Can you work these out from the model? Positions are in its coordinate system, mm. Face numbers are marked on the shaded views. A direction names the side the tool comes from. Coordinates: 2 decimals unless noted, no trailing zeros. Loops run counter-clockwise (first coordinate to the right, second up) from the corner with the lowest first, then second, coordinate; pieces in that order, holes last.
Autodesk Inventor part; units mm, degrees
ref_plane "Work Plane1" through (0, 0, 0) normal (0, 1, 0) x (1, 0, 0)
ref_plane "YZ Plane" through (0, 0, 0) normal (1, 0, 0) x (0, 1, 0)
ref_plane "XZ Plane" through (0, 0, 0) normal (0, 1, 0) x (-1, 0, 0)
sketch "Sketch1" plane through (0, 0, 0) normal (0, 1, 0) x (-1, 0, 0)
  line L0 (17.0879, 31.457) -> (-17.8371, 31.457)
  line L1 (-17.8371, 31.457) -> (-17.8371, -31.3318)
  line L2 (-17.8371, -31.3318) -> (17.0879, -31.3318)
  line L3 (17.0879, -31.3318) -> (17.0879, 31.457)
  point P0 (0, 0)
  dimension "d0" = 34.925
  dimension "d1" = 62.7888
extrude "Extrusion1" add sketch "Sketch1" along normal blind 9.7028
sketch "Sketch2" plane through (0, 9.7028, 0) normal (0, 1, 0) x (1, 0, 0)
  line L0 (17.8371, -31.457) -> (17.8371, 31.3318)
  line L1 (-17.0879, 31.3318) -> (-17.0879, -31.457)
  line L2 (17.8371, 31.3318) -> (-17.0879, 31.3318)
  line L3 (-17.0879, 31.3318) -> (-17.0879, 21.1718)
  line L4 (-17.0879, 21.1718) -> (17.8371, 21.1718)
  line L5 (17.8371, 21.1718) -> (17.8371, 31.3318)
  point P0 (0, 0)
  dimension "d4" = 10.16
extrude "Extrusion2" add sketch "Sketch2" along normal blind 11.049
sketch "Sketch3" plane through (0, 0, 0) normal (0, -1, 0) x (1, 0, 0)
  line L0 (17.8371, -31.3318) -> (-17.0879, -31.3318)
  line L1 (-17.0879, -31.3318) -> (-17.0879, -25.0072)
  line L2 (-17.0879, -31.3318) -> (-17.0879, 31.457)
  line L3 (-17.0879, -25.0072) -> (-3.5751, -25.0072)
  line L4 (-3.5751, -25.0072) -> (-3.5751, -18.962)
  line L5 (-3.5751, -18.962) -> (-3.2703, -18.962)
  line L6 (-3.2703, -18.962) -> (-3.2703, 10.883)
  line L7 (-3.2703, 10.883) -> (-3.5751, 10.883)
  line L8 (-3.5751, 10.883) -> (-3.5751, 16.9282)
  line L9 (-3.5751, 16.9282) -> (-16.9609, 16.9282)
  line L10 (-16.9609, 16.9282) -> (-17.0879, 16.9282)
  point P0 (0, 0)
  dimension "d7" = 6.3246
  dimension "d8" = 13.5128
  dimension "d9" = 6.0452
  dimension "d10" = 0.3048
  dimension "d11" = 29.845
  dimension "d14" = 0.3048
  dimension "d15" = 6.0452
  dimension "d16" = 13.3858
extrude "Extrusion3" cut sketch "Sketch3" against normal blind 2.794
sketch "Sketch4" plane through (0, 2.794, 0) normal (0, -1, 0) x (1, 0, 0)
  line L0 (-3.5751, 16.9282) -> (-17.0879, 16.9282)
  line L1 (-17.0879, 16.9282) -> (-17.0879, 10.883)
  line L2 (-17.0879, 10.883) -> (-3.5751, 10.883)
  line L3 (-3.5751, 10.883) -> (-3.5751, 16.9282)
  point P0 (0, 0)
  dimension "d19" = 13.5128
  dimension "d20" = 6.0452
sketch "Sketch5" plane through (0, 2.794, 0) normal (0, -1, 0) x (1, 0, 0)
  line L0 (-3.5751, -18.962) -> (-3.5751, -25.0072)
  line L1 (-3.5751, -25.0072) -> (-17.0879, -25.0072)
  line L2 (-17.0879, -25.0072) -> (-17.0879, -18.962)
  line L3 (-17.0879, -18.962) -> (-3.5751, -18.962)
  line L4 (-3.5751, -18.962) -> (-3.5751, -25.0072)
  point P0 (0, 0)
  dimension "d21" = 13.5128
  dimension "d22" = 6.0452
extrude "Extrusion5" add sketch "Sketch4" along normal blind 1.5748
extrude "Extrusion6" add sketch "Sketch5" along normal blind 1.5748
sketch "Sketch6" plane through (0, 9.7028, 0) normal (0, 1, 0) x (1, 0, 0)
  circle A0 centre (-11.6221, -2.8625) radius 7.9629
  line L0 (-17.0879, 18.962) -> (-17.0879, -10.883)
  line L1 (-11.6221, -10.1806) -> (-11.6221, 5.913) construction
  line L2 (-14.7946, -10.1806) -> (-14.7946, 5.913)
  line L3 (-8.4496, 5.913) -> (-8.4496, -10.1806)
  arc A1 (-8.4496, 5.913) -> (-14.7946, 5.913) centre (-11.6221, 5.913) ccw
  point P0 (0, 0)
  point P1 (-17.0879, 21.1718)
  point P2 (-11.6221, -2.1338)
  point P3 (-17.0879, 2.9283)
  point P4 (-17.0879, -8.6532)
  point P5 (-8.4496, 4.4412)
  point P6 (-14.7946, 4.4412)
  dimension "d31" = 15.9258
extrude "Extrusion7" cut sketch "Sketch6" against normal blind 25.4 contours A0 L3 | L3 A0 L2 | A0 L2 A1 L3 | L2 A0 L0
ref_plane "Work Plane1" through (0, 0, 0) normal (0, 1, 0) x (1, 0, 0)
sketch "Sketch7" plane through (0, 9.7028, 0) normal (0, 1, 0) x (1, 0, 0)
  line L0 (17.8371, -31.457) -> (17.8371, -28.663)
  line L1 (17.8371, -28.663) -> (17.8371, -26.4532)
  line L2 (14.7637, -26.4532) -> (12.5539, -26.4532)
  circle A0 centre (12.5539, -26.4532) radius 2.2098
  circle A1 centre (12.5539, -5.168) radius 2.2098
  line L3 (-17.0879, -8.6532) -> (-17.0879, -31.457)
  line L4 (-17.0879, -26.4532) -> (-13.7859, -26.4532) construction
  circle A2 centre (-11.5761, -26.4532) radius 2.2098
  line L5 (-11.5761, -14.7184) -> (-11.5761, -13.4484)
  circle A3 centre (-11.5761, -13.4484) radius 1.27
  line L6 (-11.5761, -13.4484) -> (-17.0879, -13.4484)
  line L7 (-17.0879, -16.9282) -> (-17.0879, -10.883)
  circle A4 centre (12.5539, -5.168) radius 4.1148
  circle A5 centre (12.5539, -26.4532) radius 4.1148
  circle A6 centre (-11.5761, -26.4532) radius 4.1148
  point P0 (0, 0)
  dimension "d37" = 2.794
  dimension "d38" = 2.2098
  dimension "d39" = 3.0734
  dimension "d40" = 2.2098
  dimension "d42" = 4.4196
  dimension "d43" = 4.4196
  dimension "d47" = 4.4196
  dimension "d49" = 1.27
  dimension "d50" = 2.54
  dimension "d58" = 8.2296
  dimension "d59" = 8.2296
  dimension "d60" = 8.2296
extrude "Extrusion8" cut sketch "Sketch7" against normal blind 25.4 contours A0 | A1 | A2 | A3 L6 L5 | L5 L6 A3
sketch "Sketch9" plane through (0, 1.2192, 0) normal (0, -1, 0) x (1, 0, 0)
  line L0 (-3.5751, -18.962) -> (-17.0879, -18.962)
  line L1 (-17.0879, -18.962) -> (-11.5761, -18.962)
  line L2 (-11.5761, -25.0595) -> (-11.5761, -21.2495)
  circle A0 centre (-11.5761, -21.2495) radius 1.27
  point P0 (0, 0)
  dimension "d53" = 5.5118
  dimension "d54" = 3.81
  dimension "d55" = 2.54
extrude "Extrusion9" cut sketch "Sketch9" against normal blind 8.4836
sketch "Sketch11" plane through (0, 0, 0) normal (0, -1, 0) x (1, 0, 0)
  circle A0 centre (-11.5761, 26.4532) radius 2.2098
  circle A1 centre (-11.5761, 26.4532) radius 4.1148
  circle A2 centre (12.5539, 26.4532) radius 2.2098
  circle A3 centre (12.5539, 26.4532) radius 4.1148
  circle A4 centre (12.5539, 5.168) radius 2.2098
  circle A5 centre (12.5539, 5.168) radius 4.1148
  point P0 (0, 0)
  dimension "d62" = 8.2296
  dimension "d63" = 8.2296
  dimension "d64" = 8.2296
extrude "Extrusion10" cut sketch "Sketch11" against normal blind 5.6642 contours A0 | A1 | A3 | A5
sketch "Sketch12" plane through (17.8371, 0, -31.3318) normal (0, 0, -1) x (-1, 0, 0)
  line L0 (0, 0) -> (0, 20.7518)
  line L1 (0, 20.7518) -> (13.9446, 20.7518)
  line L2 (0, 20.7518) -> (34.925, 20.7518)
  line L3 (13.9446, 20.7518) -> (17.4117, 20.7518)
  line L4 (17.4117, 20.7518) -> (17.4117, 17.9832)
  line L5 (17.4117, 17.9832) -> (17.4117, 14.5161)
  circle A0 centre (17.4117, 14.5161) radius 2.2479
  circle A1 centre (17.4117, 14.5161) radius 3.4671
  point P0 (17.8371, 0)
  dimension "d67" = 13.9446
  dimension "d68" = 3.4671
  dimension "d69" = 2.7686
  dimension "d70" = 3.4671
  dimension "d71" = 4.4958
  dimension "d72" = 6.9342
extrude "Extrusion11" cut sketch "Sketch12" against normal through all contours A0
extrude "Extrusion13" cut sketch "Sketch12" against normal blind 4.4958
sketch "Sketch13" plane through (-17.0879, 20.7518, -21.1718) normal (0, 0, 1) x (1, 0, 0)
  circle A0 centre (17.5133, -6.2357) radius 3.4671
  circle A1 centre (17.5133, -6.2357) radius 2.7813
  point P0 (17.0879, -20.7518)
  dimension "d79" = 5.5626
extrude "Extrusion14" cut sketch "Sketch13" against normal blind 4.1656 contours A0 | A1
sketch "Sketch14" plane through (0, 9.7028, 0) normal (0, 1, 0) x (1, 0, 0)
  circle A0 centre (7.9099, -5.168) radius 1.7354
  point P0 (0, 0)
extrude "Extrusion15" cut sketch "Sketch14" against normal blind 12.7
properties part number "Hand1"
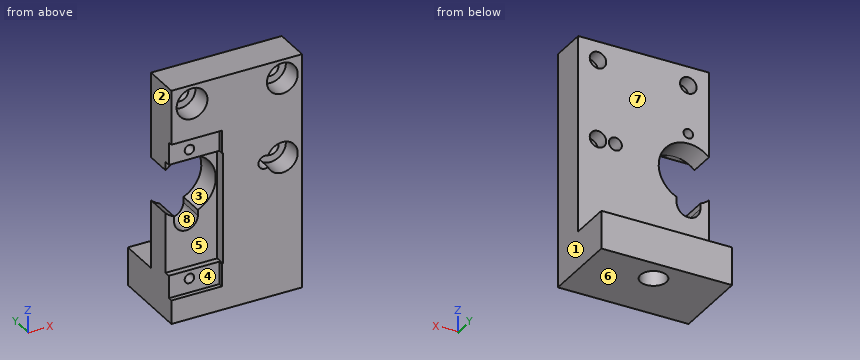
(1) Which directions (+Z, -Z, +X, -X, +Y, -Y) give clear straight access to the entire face, cutting with the end or side of a thin tool? Please do the marked faces 5, 6, 7 and 8.
Check values:
face 5: -X, -Y
face 6: -Z, +X, -X, +Y, -Y
face 7: +Z, +X, -X, +Y
face 8: +Y, -Y
(2) I want a section at A-A on y = 13.75. Write out the boundary of the cut face in (x, z).
Check values:
outline: (-17.09, -31.33) - (-2.96, -31.33) - (-2.96, -26.84) - (-1.69, -26.84) - (-1.69, -25.34) - (-2.96, -25.34) - (-2.96, -21.17) - (-17.09, -21.17) - close; (2.54, -26.84) - (3.81, -26.84) - (3.81, -31.33) - (17.84, -31.33) - (17.84, -21.17) - (3.81, -21.17) - (3.81, -25.34) - (2.54, -25.34) - close
(3) If I drill on probe 1 along Z at (x, y) = (-13, 3); probe 2 along Z at (x, y) = (8, 1.75); probe 3 along Z at (x, y) = (4, 18.25), over which ranges is the centre line in solid material (lowest first)?
Check values:
probe 1: z = -31.33 to -8.77, 10.71 to 22.59, 30.31 to 31.46
probe 2: z = -31.33 to 3.43, 6.9 to 31.46
probe 3: z = -31.33 to -21.17
(4) I want a section at D-D on y = 2. Write out the boundary of the cut face in (x, z).
Check values:
outline: (-17.09, -31.33) - (17.84, -31.33) - (17.84, 31.46) - (-17.09, 31.46) - (-17.09, 10.88) - (-3.27, 10.88) - (-3.27, -18.96) - (-17.09, -18.96) - close; hole circle Ø8.23 at (-11.58, 26.45); hole circle Ø2.54 at (-11.58, -21.25); hole circle Ø2.54 at (-11.58, 13.45); hole circle Ø8.23 at (12.55, 26.45); hole (8.73, 3.64) arc R4.11 ccw (long way) to (8.73, 6.7) arc R1.74 ccw (long way) to start
(5) I want a section at C-C on x = 13.5. Write out the boundary of the cut face in (y, z).
Check values:
outline: (0, -31.33) - (20.75, -31.33) - (20.75, -21.17) - (9.7, -21.17) - (9.7, 3.17) - (5.66, 3.17) - (5.66, 1.16) - (0, 1.16) - close; (0, 9.17) - (5.66, 9.17) - (5.66, 7.17) - (9.7, 7.17) - (9.7, 24.46) - (5.66, 24.46) - (5.66, 22.45) - (0, 22.45) - close; (0, 30.46) - (5.66, 30.46) - (5.66, 28.45) - (9.7, 28.45) - (9.7, 31.46) - (0, 31.46) - close
(6) I want a section at B-B on z = 6. Write out the boundary of the cut face in (x, y), then the cut area to 3 significant figures.
Check values:
outline: (-4.3, 2.79) - (-3.27, 2.79) - (-3.27, 0) - (6.39, 0) - (6.39, 9.7) - (-4.3, 9.7) - close; (9.43, 5.66) - (10.51, 5.66) - (10.51, 9.7) - (9.43, 9.7) - close; (14.6, 5.66) - (16.58, 5.66) - (16.58, 0) - (17.84, 0) - (17.84, 9.7) - (14.6, 9.7) - close
area: 125 mm2
(7) If we mould it in two halves opening along X, with no side actions, what happens to the marked faces 1, 2, 3 and 4? For each: released by +X, released by -X, zero draft, split by the parting line, or undercut.
Check values:
face 1: released by +X
face 2: released by -X
face 3: undercut
face 4: zero draft
(8) I'm going to push flat-ended pins straight in: pin 1 (5 mm diameter, centred on x = -7, z = -20.5, fed in from -Y); pin 2 (5.5 mm diameter, centred on x = 0, y = 16, fed in from +Z); pin 3 (1 mm diameter, centred on x = -4, y = 10, fed in from +Z); pin 4 (4 mm diameter, centred on x = -6, z = 21.5, fed in from +Y). Where does each tip first touch, or does it pass through?
Check values:
pin 1: stops at y = 1.22
pin 2: stops at z = -21.17
pin 3: stops at z = 31.46
pin 4: stops at y = 9.7
